from build123d import *

# Parameters (mm, degrees)
SKETCH_1_R      = 4
EXTRUDE_1_DEPTH = 20
SKETCH_2_R      = 1
EXTRUDE_2_DEPTH = 10


with BuildPart() as part:
    # 草图1 → 凸台-拉伸1 (new body)
    with BuildSketch(Plane(origin=(0, 0, 0), x_dir=(1, 0, 0), z_dir=(0, 1, 0))):
        with Locations(Location((0, 0, 0), (0, 0, 270))):
            Circle(SKETCH_1_R)
    extrude(amount=EXTRUDE_1_DEPTH)

    # 草图2 → 凸台-拉伸2 (add)
    with BuildSketch(Plane(origin=(0, 20, 0), x_dir=(1, 0, 0), z_dir=(0, 1, 0))):
        with Locations(Location((-2.5, 0, 0), (0, 0, 270))):
            Circle(SKETCH_2_R)
    extrude_2 = extrude(amount=EXTRUDE_2_DEPTH)

    # 镜向1: 凸台-拉伸2 across plane
    add(extrude_2.mirror(Plane(origin=(0, 0, 0), x_dir=(0, 0, 1), z_dir=(1, 0, 0))))

    # 草图4 → 旋转1 (revolve)
    with BuildSketch(Plane.XZ):
        with BuildLine():
            Line((0, 0.5), (0, -0.5))
            ThreePointArc((0, -0.5), (-0.5, 0), (0, 0.5))
        make_face()
    revolve(axis=Axis((0, 0, 0.5), (0, 0, -1)))


solid = part.part
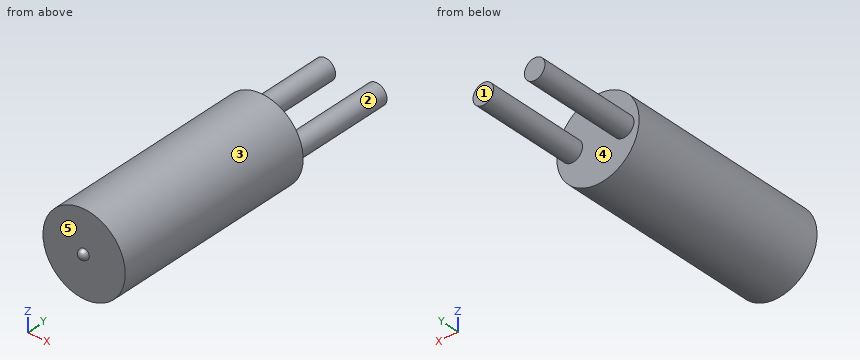
Input: part model. Units: mm. Frame: model coordinates. Face numbers are marked on the shaded views. A direction names the side the tool comes from. Coordinates: 2 decimals unless noted, no trailing zeros. Order: outer loops, then holes, each group sorted by start corner. A loop starts at its lowest first (then second) coordinate and runs counter-clockwise, first axis right, second up. Notation, with made-up numbers: M -38,-13 L -6,-13 A17 ccw -6,-6 Z; hole C 8,75.5 d4. An arc over 180 degrees is marked long. Answer in a Markdown table with one row per item.
(1) Section query C-C, the plane y = 15. Output: boundary loops of the cut face in (x, z), plus the area to 3 significant figures.
Numbers:
| item | result |
|---|---|
| outline | C 0,0 d8 |
| area | 50.3 mm^2 |
(2) Contact query for flat-ended pins moving along their axis: pin 1 Ø3 at (x, y) = (2.5, 10.5) entering from -Z; pin 2 Ø2 at (x, y) = (-3, 18.5) entering from +Z; pin 3 Ø1.5 at (x, z) = (-2, 2.5) entering from +Y; pin 4 Ø2 at (x, y) = (0, 24.5) entering from -Z. Output: stop coordinate, or through.
Numbers:
| item | result |
|---|---|
| pin 1 | stops at z = -3.87 |
| pin 2 | stops at z = 3.46 |
| pin 3 | stops at y = 20 |
| pin 4 | passes through |
(3) Section query A-A, the plane z = 0. Output: boundary loops of the cut face in (x, y).
Numbers:
| item | result |
|---|---|
| outline | M -4,0 L -0.5,0 A0.5 ccw 0.5,0 L 4,0 L 4,20 L 3.5,20 L 3.5,30 L 1.5,30 L 1.5,20 L -1.5,20 L -1.5,30 L -3.5,30 L -3.5,20 L -4,20 Z |
(4) Access query for the marked faces 1 and 2. Directions: +Z, -Z, +X, -X, +Y, -Y. A direction counts if a zero-diameter tool reaches every point of the face in a straight line with its end or side. Return the directions, or none.
Numbers:
| item | result |
|---|---|
| face 1 | +Z, -Z, +X, -X, +Y |
| face 2 | +Y |
(5) Draft query along X for the marked faces 3, 4 and 5. Return one class per face: pulls with the +X half, pulls with the -X half, needs draft (parallel to the pull), parting line crosses it, or undercut.
Numbers:
| item | result |
|---|---|
| face 3 | parting line crosses it |
| face 4 | undercut |
| face 5 | needs draft |
(6) Section query D-D, the plane x = -3. Output: boundary loops of the cut face in (y, z).
Numbers:
| item | result |
|---|---|
| outline | M 0,-2.65 L 20,-2.65 L 20,-0.87 L 30,-0.87 L 30,0.87 L 20,0.87 L 20,2.65 L 0,2.65 Z |
(7) Section query B-B, the plane x = 0. Output: boundary loops of the cut face in (y, z), plus the area to 3 significant figures.
Numbers:
| item | result |
|---|---|
| outline | M 0,-4 L 20,-4 L 20,4 L 0,4 L 0,0.5 A0.5 ccw 0,-0.5 Z |
| area | 160 mm^2 |
(8) Material intervals for line 1 (Y direction, x = -2.25, z = 0.25); line 2 (Y direction, x = 1, z = 3.5); line 3 (Z direction, x = -1, y = 14), sorted ascending. Write a range as [from, to].
Numbers:
| item | result |
|---|---|
| line 1 | y = [0, 30] |
| line 2 | y = [0, 20] |
| line 3 | z = [-3.87, 3.87] |
